Read the model definition and answer for the solid it produces. Units are mm, in the model's axes. A direction names the side the tool comes from. Round coordinates to 2 decimals unless told otherwise and drop trailing zeros. Loops run counter-clockwise (first coordinate to the right, second up) from the corner with the lowest first, then second, coordinate; pieces in that order, holes last. Notation, with made-up numbers: M 75.5,-4.5 L 98.5,-4.5 A16 ccw 98.5,24.5 Z; hole C -12,24 d1. An arc over 180 degrees is marked long. Write each question's results on one line, items separated by ' | '.
Autodesk Inventor part; units mm, degrees
ref_plane "YZ Plane" through (0, 0, 0) normal (1, 0, 0) x (0, 1, 0)
ref_plane "XZ Plane" through (0, 0, 0) normal (0, 1, 0) x (-1, 0, 0)
ref_plane "XY Plane" through (0, 0, 0) normal (0, 0, 1) x (1, 0, 0)
sketch "Sketch1" plane through (0, 0, 0) normal (0, 1, 0) x (-1, 0, 0)
  line L0 (32, 32) -> (0, 32)
  line L1 (0, 32) -> (0, 0)
  line L2 (0, 0) -> (32, 0)
  line L3 (32, 0) -> (32, 32)
extrude "Extrusion1" add sketch "Sketch1" along normal blind 55
sketch "Sketch3" plane through (-32, 0, 32) normal (0, 0, 1) x (1, 0, 0)
  line L0 (3.5, 49) -> (28.5, 49)
  line L1 (28.5, 49) -> (28.5, 31)
  line L2 (28.5, 31) -> (3.5, 31)
  line L3 (3.5, 31) -> (3.5, 49)
  line L4 (3.5, 49) -> (3.5, 43.25)
  line L5 (3.5, 36.75) -> (3.5, 43.25)
  line L6 (28.5, 49) -> (28.5, 43.25)
  line L7 (28.5, 36.75) -> (28.5, 43.25)
  line L8 (3.5, 43.25) -> (3.5, 36.75)
  line L9 (28.5, 43.25) -> (28.5, 36.75)
  point P0 (32, 0)
extrude "Extrusion3" cut sketch "Sketch3" against normal blind 2.5
sketch "Sketch4" plane through (-32, 0, 29.5) normal (0, 0, 1) x (1, 0, 0)
  line L0 (3.5, 49) -> (28.5, 49)
  line L1 (3.5, 49) -> (3.5, 43.25)
  line L2 (28.5, 31) -> (3.5, 31)
  line L3 (3.5, 36.75) -> (3.5, 31)
  line L4 (3.5, 31) -> (28.5, 31)
  line L5 (28.5, 31) -> (28.5, 36.75)
  line L6 (28.5, 49) -> (28.5, 31)
  line L7 (28.5, 43.25) -> (28.5, 49)
  line L8 (28.5, 49) -> (3.5, 49)
  point P0 (32, 0)
sketch "Sketch5" plane through (-32, 0, 29.5) normal (0, 0, 1) x (1, 0, 0)
  line L0 (3.5, 43.25) -> (8.5, 43.25)
  line L1 (8.5, 43.25) -> (8.5, 36.75)
  line L2 (8.5, 36.75) -> (3.5, 36.75)
  line L3 (3.5, 36.75) -> (3.5, 43.25)
  point P0 (32, 0)
sketch "Sketch6" plane through (-32, 0, 29.5) normal (0, 0, 1) x (1, 0, 0)
  line L0 (28.5, 43.25) -> (23.5, 43.25)
  line L1 (23.5, 43.25) -> (23.5, 36.75)
  line L2 (23.5, 36.75) -> (28.5, 36.75)
  line L3 (28.5, 36.75) -> (28.5, 43.25)
  point P0 (32, 0)
extrude "Extrusion4" cut sketch "Sketch5" against normal blind 2
extrude "Extrusion5" cut sketch "Sketch6" against normal blind 2
sketch "Sketch7" plane through (-32, 0, 29.5) normal (0, 0, 1) x (1, 0, 0)
  line L0 (3.5, 43.25) -> (8.5, 43.25)
  line L1 (3.5, 43.25) -> (3.5, 49)
  line L2 (8.5, 43.25) -> (3.5, 43.25)
  line L3 (3.5, 43.25) -> (3.5, 49)
  line L4 (3.5, 49) -> (8.5, 49)
  line L5 (8.5, 49) -> (8.5, 43.25)
  point P0 (32, 0)
sketch "Sketch8" plane through (-32, 0, 29.5) normal (0, 0, 1) x (1, 0, 0)
  line L0 (8.5, 36.75) -> (3.5, 36.75)
  line L1 (28.5, 31) -> (3.5, 31)
  line L2 (8.5, 36.75) -> (3.5, 36.75)
  line L3 (3.5, 36.75) -> (3.5, 31)
  line L4 (3.5, 31) -> (8.5, 31)
  line L5 (8.5, 31) -> (8.5, 36.75)
  point P0 (32, 0)
sketch "Sketch9" plane through (-32, 0, 29.5) normal (0, 0, 1) x (1, 0, 0)
  line L0 (28.5, 36.75) -> (23.5, 36.75)
  line L1 (28.5, 31) -> (3.5, 31)
  line L2 (23.5, 36.75) -> (28.5, 36.75)
  line L3 (28.5, 36.75) -> (28.5, 31)
  line L4 (28.5, 31) -> (23.5, 31)
  line L5 (23.5, 31) -> (23.5, 36.75)
  point P0 (32, 0)
sketch "Sketch10" plane through (-32, 0, 29.5) normal (0, 0, 1) x (1, 0, 0)
  line L0 (23.5, 43.25) -> (28.5, 43.25)
  line L1 (28.5, 49) -> (28.5, 43.25)
  line L2 (23.5, 43.25) -> (28.5, 43.25)
  line L3 (28.5, 43.25) -> (28.5, 49)
  line L4 (28.5, 49) -> (23.5, 49)
  line L5 (23.5, 49) -> (23.5, 43.25)
  point P0 (32, 0)
extrude "Extrusion6" add sketch "Sketch7" along normal blind 1
extrude "Extrusion7" add sketch "Sketch8" along normal blind 1
extrude "Extrusion8" add sketch "Sketch9" along normal blind 1
extrude "Extrusion9" add sketch "Sketch10" along normal blind 1
sketch "Sketch11" plane through (-32, 0, 30.5) normal (0, 0, 1) x (1, 0, 0)
  line L0 (23.5, 43.25) -> (28.5, 43.25)
  line L1 (23.5, 43.25) -> (25, 43.25)
  line L2 (25, 43.25) -> (25, 44.25)
  line L3 (25, 44.25) -> (23.5, 44.25)
  line L4 (23.5, 44.25) -> (23.5, 43.25)
  point P0 (32, 0)
extrude "Extrusion10" cut sketch "Sketch11" against normal blind 1
sketch "Sketch12" plane through (-32, 0, 29.5) normal (0, 0, 1) x (1, 0, 0)
  line L0 (8.5, 49) -> (8.5, 43.25)
  line L1 (23.5, 31) -> (8.5, 31)
  line L2 (23.5, 49) -> (23.5, 44.25)
  point P0 (32, 0)
sketch "Sketch13" plane through (-32, 0, 29.5) normal (0, 0, 1) x (1, 0, 0)
  point P0 (32, 0)
sketch "Sketch14" plane through (-32, 0, 29.5) normal (0, 0, 1) x (1, 0, 0)
  line L0 (23.5, 44.25) -> (23.5, 49)
  line L1 (23.5, 49) -> (17.5, 49)
  line L2 (14.5, 43) -> (17.5, 43)
  line L3 (17.5, 38) -> (18, 38)
  line L4 (18, 38) -> (18, 43)
  line L5 (18, 43) -> (14, 43)
  line L6 (14, 43) -> (14, 38)
  line L7 (14, 38) -> (14.5, 38)
  line L8 (14.5, 38) -> (14.5, 42)
  line L9 (3.5, 43.25) -> (8.5, 43.25)
  line L10 (14.5, 42) -> (14.5, 42.5)
  line L11 (14.5, 42.5) -> (17.5, 42.5)
  line L12 (17.5, 42.5) -> (17.5, 38)
  point P0 (32, 0)
extrude "Extrusion11" add sketch "Sketch14" along normal blind 1
sketch "Sketch15" plane through (-32, 0, 29.5) normal (0, 0, 1) x (1, 0, 0)
  line L0 (14.5, 42.5) -> (14.5, 38)
  line L1 (14.5, 42.5) -> (17.5, 42.5)
  line L2 (17.5, 42.5) -> (17.5, 39.5)
  line L3 (17.5, 39.5) -> (14.5, 39.5)
  line L4 (14.5, 39.5) -> (14.5, 42.5)
  point P0 (32, 0)
extrude "Extrusion12" cut sketch "Sketch15" against normal blind 8.5
sketch "Sketch16" plane through (-32, 0, 32) normal (0, 0, 1) x (1, 0, 0)
  point P0 (32, 0)
sketch "Sketch17" plane through (0, 0, 32) normal (1, 0, 0) x (0, 0, -1)
  line L0 (2, 46) -> (20, 46)
  line L1 (20, 46) -> (20, 8)
  line L2 (20, 8) -> (2, 8)
  line L3 (2, 8) -> (2, 46)
  point P0 (32, 0)
extrude "Extrusion13" cut sketch "Sketch17" against normal blind 1.5
sketch "Sketch18" plane through (-1.5, 0, 32) normal (1, 0, 0) x (0, 0, -1)
  line L0 (20, 38.5) -> (14, 38.5)
  line L1 (14, 38.5) -> (14, 46)
  line L2 (14, 46) -> (20, 46)
  line L3 (20, 46) -> (20, 38.5)
  point P0 (32, 0)
extrude "Extrusion14" cut sketch "Sketch18" against normal blind 9.5
sketch "Sketch19" plane through (0, 55, 0) normal (0, 1, 0) x (1, 0, 0)
  circle A0 centre (-16, -16) radius 10.5
  point P0 (0, 0)
sketch "Sketch20" plane through (0, 55, 0) normal (0, 1, 0) x (1, 0, 0)
  point P0 (0, 0)
extrude "Extrusion15" cut sketch "Sketch19" against normal blind 2
sketch "Sketch21" plane through (-32, 0, 0) normal (-1, 0, 0) x (0, 0, 1)
  line L0 (32, 0) -> (32, 55)
  line L1 (0, 0) -> (32, 0)
  line L2 (32, 0) -> (32, 55)
  line L3 (32, 55) -> (0, 55)
  line L4 (0, 55) -> (0, 0)
extrude "Extrusion16" add sketch "Sketch21" along normal blind 4
sketch "Sketch22" plane through (-36, 0, 0) normal (-1, 0, 0) x (0, 0, 1)
  line L0 (2, 3) -> (4, 3)
  line L1 (4, 3) -> (4, 52)
  line L2 (4, 52) -> (2, 52)
  line L3 (2, 52) -> (2, 3)
  line L4 (23, 3) -> (25, 3)
  line L5 (25, 3) -> (25, 52)
  line L6 (25, 52) -> (23, 52)
  line L7 (23, 52) -> (23, 3)
  point P0 (0, 0)
extrude "Extrusion17" cut sketch "Sketch22" against normal blind 11
sketch "Sketch24" plane through (-16, 53, 16) normal (0, 1, 0) x (1, 0, 0)
  line L0 (-5.1, 5.1) -> (5.1, 5.1)
  line L1 (5.1, 5.1) -> (5.1, -5.1)
  line L2 (5.1, -5.1) -> (-5.1, -5.1)
  line L3 (-5.1, -5.1) -> (-5.1, 5.1)
  point P0 (16, 16)
extrude "Extrusion19" cut sketch "Sketch24" against normal blind 28
properties part number "Cuvette Holder v2_3DPrint"
Item 1: Straight lines are drawn through the part: line 1 (Z direction, x = -33, y = 23.5); line 2 (Y direction, x = -10, z = 30); line 3 (Z direction, x = -16, y = 54). For each, find the intervals that lie inside material, in ascending order.
Outcome:
line 1: z = 0 to 2, 4 to 23, 25 to 32 | line 2: y = 0 to 31, 49 to 55 | line 3: z = 0 to 5.5, 26.5 to 32
Item 2: Flat-ended cylindrical pins translate along their axes: pin 1 (2.5 mm diameter, centred on x = -5.5, y = 41.5, fed in from +Z); pin 2 (5 mm diameter, centred on y = 40, z = 15, fed in from +X); pin 3 (10 mm diameter, centred on x = -12, z = 12.5, fed in from +Y). Find the tip coordinate at first contact, or state that the pin passes through.
Outcome:
pin 1: stops at z = 27.5 | pin 2: stops at x = -1.5 | pin 3: stops at y = 53
Item 3: The part is cut by section D-D (y = 26). Determine the outline of the cut face in (x, z).
Outcome:
outline: M -36,0 L 0,0 L 0,12 L -1.5,12 L -1.5,30 L 0,30 L 0,32 L -36,32 L -36,25 L -25,25 L -25,23 L -36,23 L -36,4 L -25,4 L -25,2 L -36,2 Z; hole M -21.1,10.9 L -10.9,10.9 L -10.9,21.1 L -21.1,21.1 Z
Item 4: The part is cut by section C-C (x = -31.5). Determine the outline of the cut face in (y, z), plus the area to 3 significant figures.
Outcome:
outline: M 0,0 L 55,0 L 55,32 L 0,32 Z; hole M 3,2 L 52,2 L 52,4 L 3,4 Z; hole M 3,23 L 52,23 L 52,25 L 3,25 Z | area: 1,560 mm2
Item 5: The mould has two halves that part along Y. Classify faces 5 (the face through (-23.5, 40, 29)), 6 (the face through (-18, 0, 16)), 7 (the face through (-36, 28, 16)): pulls with the +Y half, pulls with the -Y half, needs draft (parallel to the pull), parting line crosses it, or undercut.
Outcome:
face 5: undercut | face 6: pulls with the -Y half | face 7: needs draft
Item 6: The part is cut by section A-A (z = 16). Determine the outline of the cut face in (x, y), plus the area to 3 significant figures.
Outcome:
outline: M -36,0 L 0,0 L 0,8 L -1.5,8 L -1.5,38.5 L -10.9,38.5 L -10.9,25 L -21.1,25 L -21.1,53 L -26.5,53 L -26.5,55 L -36,55 Z; M -10.9,46 L 0,46 L 0,55 L -5.5,55 L -5.5,53 L -10.9,53 Z | area: 1,520 mm2
Item 7: The part is cut by section B-B (x = -16). Determine the outline of the cut face in (y, z), plus the area to 3 significant figures.
Outcome:
outline: M 0,0 L 55,0 L 55,5.5 L 53,5.5 L 53,10.9 L 25,10.9 L 25,21.1 L 39.5,21.1 L 39.5,29.5 L 31,29.5 L 31,32 L 0,32 Z; M 42.5,21.1 L 53,21.1 L 53,26.5 L 55,26.5 L 55,32 L 49,32 L 49,29.5 L 43,29.5 L 43,30.5 L 42.5,30.5 Z | area: 1,360 mm2
Item 8: For faces 1 (the face through (-31, 27, 25)), 2 (the face through (-16, 39, 21.1)), 3 (the face through (0, 27, 9)), 4 (the face through (-14.5, 41, 26)), determine the directions among +Z, -Z, +X, -X, +Y, -Y from which every point of the face is accessible in a straight line to the end or side of a thin tool.
Outcome:
face 1: -X | face 2: +Y | face 3: +Z, -Z, +X, +Y, -Y | face 4: +Z
